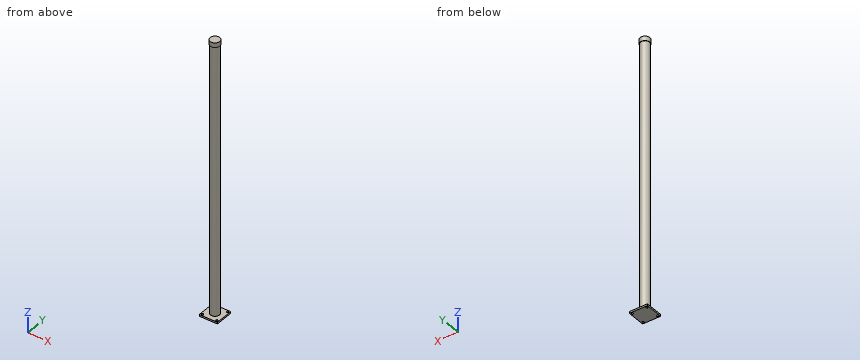
```python
from build123d import *

# Parameters (mm, degrees)
F0_R     = 25.4
F0_R_2   = 22.225
F1_DEPTH = 1524
F2_W     = 101.6
F2_H     = 101.6
F2_R     = 5.489771
F3_DEPTH = 9.525
F4_R     = 26.792936
F5_DEPTH = 25.4


with BuildPart() as f1:
    # F0 (on Top) → F1 (new body)
    with BuildSketch(Plane.XY):
        Circle(F0_R)
        Circle(F0_R_2, mode=Mode.SUBTRACT)
    extrude(amount=F1_DEPTH)

    # F2 (on Top) → F3 (join)
    with BuildSketch(Plane.XY):
        Rectangle(F2_W, F2_H)
        with Locations((-40.11862, -40.534951)):
            Circle(F2_R, mode=Mode.SUBTRACT)
        with Locations((40.11862, -40.534951)):
            Circle(F2_R, mode=Mode.SUBTRACT)
        with Locations((-40.11862, 40.534951)):
            Circle(F2_R, mode=Mode.SUBTRACT)
        with Locations((40.11862, 40.534951)):
            Circle(F2_R, mode=Mode.SUBTRACT)
    extrude(amount=-F3_DEPTH)

    # F4 (on face) → F5 (join)
    with BuildSketch(Plane.XY.offset(1524)):
        Circle(F4_R)
    extrude(amount=-F5_DEPTH)


solid = f1.part
```
Here's how the part is built. I have some questions about the finished solid (model axes, mm). Give positions to 0.01 mm unless a question says otherwise; leave off trailing zeros. Write each loop counter-clockwise with the first axis right and the second up, starting at its lowest first coordinate (ties: lowest second). Pieces come first, ordered by that corner, then holes. Notation, with made-up numbers: M 81.5,54 L 131.5,54 A22 ccw 131.5,75 Z; hole C 27,26 d11. An arc over 180 degrees is marked long. Put each result on its own line as item: value. Start each with the question number.
Item 1: I need wall thicknesses on L1, parallel to Y at x = 1, z = 61.5; L2, parallel to X at y = 0, z = 719 (3 decimals); L3, parallel to X at y = 20.5, z = 1297.5. Which ranges of each line are inside material? Lowest first, please. Write a range as from..to.
Item 2: If we section it at A-A, the plane x = 0: Write out the boundary of the cut face in (y, z) (3 decimals).
Item 3: Will these pins go through, and if not, where does the flat tip stop? pin 1 (3 mm diameter, centred on x = 12.5, y = 25.5, fed in from +Z); pin 2 (3 mm diameter, centred on x = 21, z = 486.5, fed in from +Y); pin 3 (1 mm diameter, centred on y = 18.5, z = 945.5, fed in from -X).
Item 4: If we section it at C-C, the plane z = 160: Write out the boundary of the cut face in (x, y) (3 decimals).
Values:
1. L1: -25.38..-22.2, 22.2..25.38
1. L2: -25.4..-22.225, 22.225..25.4
1. L3: -15..-8.58, 8.58..15
2. outline: M -50.8,-9.525 L 50.8,-9.525 L 50.8,0 L 25.4,0 L 25.4,1498.6 L 26.793,1498.6 L 26.793,1524 L -26.793,1524 L -26.793,1498.6 L -25.4,1498.6 L -25.4,0 L -50.8,0 Z; hole M -22.225,0 L 22.225,0 L 22.225,1498.6 L -22.225,1498.6 Z
3. pin 1: z = 0
3. pin 2: y = 16.28
3. pin 3: x = -17.92
4. outline: C 0,0 d50.8; hole C 0,0 d44.45
